For this review, take the finished solid that the model builds, in its own axes (mm). Face numbers are marked on the shaded views. A direction names the side the tool comes from. Give positions to 0.01 mm unless a question says otherwise; leave off trailing zeros. Write each loop counter-clockwise with the first axis right and the second up, starting at its lowest first coordinate (ties: lowest second). Pieces come first, ordered by that corner, then holes.
from build123d import *

# Parameters (mm, degrees)
SKETCH1_R           = 17.5
SKETCH1_R_2         = 2
BOSS_EXTRUDE1_DEPTH = 4
SKETCH2_R           = 7.5
SKETCH2_R_2         = 4
BOSS_EXTRUDE2_DEPTH = 10


with BuildPart() as part:
    # Sketch1 → Boss-Extrude1 (new body)
    with BuildSketch(Plane(origin=(0, 0, 0), x_dir=(1, 0, 0), z_dir=(0, 1, 0))):
        Circle(SKETCH1_R)
        with Locations((0, 12.5)):
            Circle(SKETCH1_R_2, mode=Mode.SUBTRACT)
        with Locations((0, -12.5)):
            Circle(SKETCH1_R_2, mode=Mode.SUBTRACT)
    extrude(amount=BOSS_EXTRUDE1_DEPTH)

    # Sketch2 → Boss-Extrude2 (add)
    with BuildSketch(Plane(origin=(0, 4, 0), x_dir=(1, 0, 0), z_dir=(0, 1, 0))):
        Circle(SKETCH2_R)
        Circle(SKETCH2_R_2, mode=Mode.SUBTRACT)
    extrude(amount=BOSS_EXTRUDE2_DEPTH)


solid = part.part
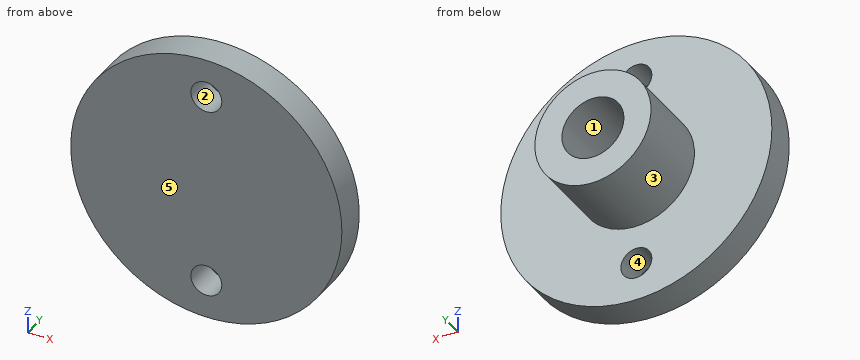
(1) We need section D-D (y = 1.5). Write out the cut boundary in (x, z), and give its area (3 significant figures).
(2) Clearance check with flat-ended pins moving along their axes: pin 1 Ø5 at (x, z) = (8.5, 3) entering from -Y; pin 2 Ø2 at (x, z) = (-4, 9) entering from +Y; pin 3 Ø6 at (y, z) = (6, -3) entering from -X; pin 4 Ø1 at (y, z) = (3.5, 10.5) entering from -X. State where each tip first meets the part, or that it passes through.
(3) We need section C-C (z = 0). Write out the cut boundary in (x, y).
(4) Tool access review of the marked faces 1 and 2: name each direction out of +Z, -Z, +X, -X, +Y, -Y from which nothing blocks a thin tool from reaching the whole face with its end or side.
(5) We need section A-A (x = 0). Write out the cut boundary in (y, z), and give its area (3 significant figures).
(6) We need section B-B (z = -12.5). Write out the cut boundary in (x, y), and give its area (3 significant figures).
(7) For L1, parallel to Z at x = 0, y = 2; L2, parallel to X at y = 8.5, z = 0, list the stretches that pass through material, from the lowest coordinate up.
(8) The part is to be moulded in two halves that separate along X. For the marked faces 3, 4 and 5, say which applies: +X half, -X half, draft (parallel to the pull), parting line (faces both ways), or undercut.
The answers:
1. outline: circle Ø35 at (0, 0); hole circle Ø4 at (0, -12.5); hole circle Ø4 at (0, 12.5)
1. area: 937 mm2
2. pin 1: stops at y = 0
2. pin 2: stops at y = 4
2. pin 3: stops at x = -17.48
2. pin 4: stops at x = -14.36
3. outline: (-17.5, 0) - (17.5, 0) - (17.5, 4) - (7.5, 4) - (7.5, 14) - (4, 14) - (4, 4) - (-4, 4) - (-4, 14) - (-7.5, 14) - (-7.5, 4) - (-17.5, 4) - close
4. face 1: +Y
4. face 2: +Y, -Y
5. outline: (0, -17.5) - (4, -17.5) - (4, -14.5) - (0, -14.5) - close; (0, -10.5) - (4, -10.5) - (4, -7.5) - (14, -7.5) - (14, -4) - (4, -4) - (4, 4) - (14, 4) - (14, 7.5) - (4, 7.5) - (4, 10.5) - (0, 10.5) - close; (0, 14.5) - (4, 14.5) - (4, 17.5) - (0, 17.5) - close
5. area: 178 mm2
6. outline: (-12.25, 0) - (-2, 0) - (-2, 4) - (-12.25, 4) - close; (2, 0) - (12.25, 0) - (12.25, 4) - (2, 4) - close
6. area: 82.0 mm2
7. L1: z = -17.5 to -14.5, -10.5 to 10.5, 14.5 to 17.5
7. L2: x = -7.5 to -4, 4 to 7.5
8. face 3: parting line
8. face 4: undercut
8. face 5: draft
